Build history of the part. All positions in model axes, mm. A direction names the side the tool comes from. Round coordinates to 2 decimals unless told otherwise and drop trailing zeros. Loops run counter-clockwise (first coordinate to the right, second up) from the corner with the lowest first, then second, coordinate; pieces in that order, holes last. Notation, with made-up numbers: (77.25, 64.5) -> (124.25, 64.5) arc R27 ccw to (124.25, 93.5) -> close; hole circle Ø11 at (53.25, 88). An arc over 180 degrees is marked (long way). Put each result on its own line as item: value. Start each with the question number.
Item 1: Cut at C-C, the plane y = 16.5. List the corners of the cut face in (x, z) (3 decimals), plus the area to 3 significant figures.
Item 2: Pull direction Z, two halves, no side cores. Call faces 3 (the flat face through (41.275, 12, 1)), 4 (the cylindrical face through (-23.73, 25.1, -23.34)), 5 (the flat face through (-1, 12, -41.275)): +Z half, -Z half, draft (parallel to the pull), parting line (faces both ways), or undercut.
Item 3: Drill centre lines: probe 1 along X at (y, z) = (14, 32) (3 decimals); probe 2 along Z at (x, y) = (34, 14) (3 decimals); probe 3 along Y at (x, z) = (-32.5, 20). Where is each one in solid material? Low to high. Write a range as [from, to].
Item 4: Tool access for faces 1 (the flat face through (-38, 18.263, 33)), 2 (the flat face through (-1, 12, 41.275)): list every direction of +Z, -Z, +X, -X, +Y, -Y with a clear straight run to the whole face (end or side of a thin tool).
Item 5: Cut at A-A, the plane z = 0. List the corners of the cut face in (x, y) (3 decimals).
Item 6: Cut at B-B, the plane y = 29. List the corners of the cut face in (x, z) (3 decimals).
Item 7: Flat gauge pins, fed straight in: pin 1 Ø12 at (x, z) = (30.96, 30.96) entering from +Y; pin 2 Ø6 at (x, z) = (-26, 27) entering from +Y. Where does each tip first touch, or does it go through?
```python
from build123d import *

# Parameters (mm, degrees)
SKETCH1_W          = 82.55
SKETCH1_H          = 82.55
SKETCH1_R          = 30.9753
EXTRUDE1_DEPTH     = 31.75
CUT_EXTRUDE1_DEPTH = 13.4874
HOLE1_D            = 13.4874
HOLE1_DEPTH        = 18.2626


with BuildPart() as part:
    # Sketch1 → Extrude1 (new body)
    with BuildSketch(Plane(origin=(0, 0, 0), x_dir=(1, 0, 0), z_dir=(0, 1, 0))):
        Rectangle(SKETCH1_W, SKETCH1_H)
        with Locations(Location((0, 0, 0), (0, 0, 270))):  # turned: the seam where the file's is
            Circle(SKETCH1_R, mode=Mode.SUBTRACT)
    extrude(amount=EXTRUDE1_DEPTH)

    # Sketch2 → Cut-Extrude1 (cut)
    with BuildSketch(Plane(origin=(0, 31.75, 0), x_dir=(1, 0, 0), z_dir=(0, 1, 0))):
        with BuildLine():
            Line((23.319621037, -41.275), (41.275, -41.275))
            Line((41.275, -41.275), (41.275, -23.319621037))
            ThreePointArc((41.275, -23.319621037), (23.531743879, -23.531743879), (23.319621037, -41.275))
        make_face()
        with BuildLine():
            Line((41.275, 41.275), (41.275, 23.319621037))
            ThreePointArc((41.275, 23.319621037), (23.531743879, 23.531743879), (23.319621037, 41.275))
            Line((23.319621037, 41.275), (41.275, 41.275))
        make_face()
        with BuildLine():
            Line((-23.319621037, 41.275), (-41.275, 41.275))
            Line((-41.275, 41.275), (-41.275, 23.319621037))
            ThreePointArc((-41.275, 23.319621037), (-23.531743879, 23.531743879), (-23.319621037, 41.275))
        make_face()
        with BuildLine():
            Line((-41.275, -41.275), (-41.275, -23.319621037))
            ThreePointArc((-41.275, -23.319621037), (-23.531743879, -23.531743879), (-23.319621037, -41.275))
            Line((-23.319621037, -41.275), (-41.275, -41.275))
        make_face()
    extrude(amount=-CUT_EXTRUDE1_DEPTH, mode=Mode.SUBTRACT)

    # Hole1
    with Locations(Plane(origin=(0, 18.2626, 0), x_dir=(-1, 0, 0), z_dir=(0, 1, 0))):
        with Locations((30.9626, 30.9626), (30.9626, -30.9626), (-30.9626, 30.9626), (-30.9626, -30.9626)):
            Hole(HOLE1_D / 2, depth=HOLE1_DEPTH)

    # Sketch5 → Cut-Revolve1 (revolve, cut)
    with BuildSketch(Plane(origin=(0, 0, 0), x_dir=(0, 0, -1), z_dir=(1, 0, 0)), mode=Mode.PRIVATE) as cut_revolve1_sk:
        Polygon((-32.131, 31.75), (-30.9753, 31.75), (-30.9753, 30.5943), align=None)
        Polygon((-30.9753, 1.1557), (-32.131, 0), (-30.9753, 0), align=None)
    revolve(cut_revolve1_sk.sketch.rotate(Axis((0, 0, 0), (0, 1, 0)), 180), axis=Axis((0, 0, 0), (0, 1, 0)), mode=Mode.SUBTRACT)  # turned: the seam where the file's is


solid = part.part
```
Reply:
1. outline: (-41.275, -41.275) -> (41.275, -41.275) -> (41.275, 41.275) -> (-41.275, 41.275) -> close; hole circle Ø13.487 at (-30.963, -30.963); hole circle Ø13.487 at (-30.963, 30.963); hole circle Ø61.951 at (0, 0); hole circle Ø13.487 at (30.963, -30.963); hole circle Ø13.487 at (30.963, 30.963)
1. area: 3,230 mm^2
2. face 3: draft
2. face 4: undercut
2. face 5: -Z half
3. probe 1: x = [-41.275, -37.626], [-24.299, 24.299], [37.626, 41.275]
3. probe 2: z = [-41.275, -36.984], [-24.942, 24.942], [36.984, 41.275]
3. probe 3: y = [0, 18.26]
4. face 1: +Y
4. face 2: +Z, +X, -X, +Y, -Y
5. outline: (-41.275, 0) -> (-32.131, 0) -> (-30.975, 1.156) -> (-30.975, 30.594) -> (-32.131, 31.75) -> (-41.275, 31.75) -> close; (30.975, 1.156) -> (32.131, 0) -> (41.275, 0) -> (41.275, 31.75) -> (32.131, 31.75) -> (30.975, 30.594) -> close
6. outline: (-41.275, -23.32) arc R12.7 cw to (-23.32, -41.275) -> (23.32, -41.275) arc R12.7 cw to (41.275, -23.32) -> (41.275, 23.32) arc R12.7 cw to (23.32, 41.275) -> (-23.32, 41.275) arc R12.7 cw to (-41.275, 23.32) -> close; hole circle Ø61.951 at (0, 0)
7. pin 1: passes through
7. pin 2: stops at y = 18.26
